For this review, take the finished solid that the model builds, in its own axes (mm). Face numbers are marked on the shaded views. A direction names the side the tool comes from. Give positions to 0.01 mm unless a question says otherwise; leave off trailing zeros. Order: outer loops, then holes, each group sorted by start corner. A loop starts at its lowest first (then second) coordinate and runs counter-clockwise, first axis right, second up. Notation, with made-up numbers: (71.5, 48) -> (101.5, 48) arc R23 ccw to (101.5, 86) -> close; hole circle Ø1 at (7, 15.25). An arc over 180 degrees is marked (long way). Use CSV: the item, a comma, the result in double quotes. Start each with the question number.
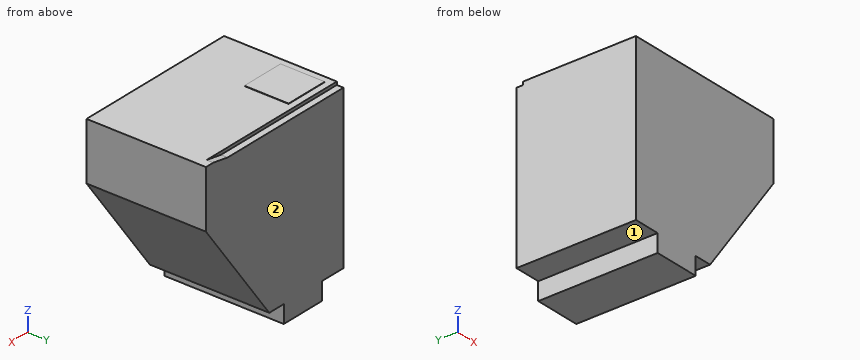
Solid Edge part; units mm, degrees
sketch "Sketch1" plane through (33.766, 0, 12.7127) normal (0, -1, 0) x (1, 0, 0)
  line L0 (-12.25, 0.75) -> (-21, -11.25)
  line L1 (-12.25, 7.25) -> (-12.25, 0.75)
  line L2 (-31.25, 7.25) -> (-12.25, 7.25)
  line L3 (-31.25, 7.25) -> (-31.25, -11.25)
  line L4 (-31.25, -11.25) -> (-28.25, -11.25)
  line L5 (-28.25, -11.25) -> (-28.25, -13.25)
  line L6 (-28.25, -13.25) -> (-23, -13.25)
  line L7 (-23, -13.25) -> (-23, -11.25)
  line L8 (-23, -11.25) -> (-21, -11.25)
extrude "Protrusion1" add sketch "Sketch1" along normal blind 13.5
sketch "Sketch2" plane through (12.016, -6.75, 19.9627) normal (0, 0, 1) x (1, 0, 0)
  line L0 (-9.5, 6.75) -> (6.5, 6.75)
  line L1 (6.5, 6.75) -> (6.5, 6)
  line L2 (6.5, 6) -> (-9.5, 6)
  line L3 (-9.5, 6) -> (-9.5, 6.75)
extrude "ExtrudedCutout_1" cut sketch "Sketch2" against normal blind 0.35
sketch "Sketch3" plane through (12.016, 0, 9.7127) normal (0, 1, 0) x (-1, 0, 0)
  line L0 (-8.5, 10.25) -> (-6.5, 9.9)
  line L1 (-6.5, 9.9) -> (-6.5, 10.25)
  line L2 (-6.5, 10.25) -> (-8.5, 10.25)
extrude "ExtrudedCutout_2" cut sketch "Sketch3" against normal blind 0.75
sketch "Sketch4" plane through (12.016, -6.75, 19.9627) normal (0, 0, 1) x (0, -1, 0)
  line L0 (-5.25, -8.75) -> (-5.25, -3.75)
  line L1 (-5.25, -3.75) -> (-0.25, -3.75)
  line L2 (-0.25, -3.75) -> (-0.25, -8.75)
  line L3 (-0.25, -8.75) -> (-5.25, -8.75)
extrude "ExtrudedProtrusion_2" add sketch "Sketch4" along normal blind 0.035
properties material "Stainless Steel, 420"
1. Clearance check with flat-ended pins moving along their axes: P1, Ø1, axis at y = -5.5, z = 0.5, coming from the +X side; P2, Ø0.6, axis at y = -6.5, z = 0, coming from the -X side; P3, Ø1.6, axis at x = 12, y = -9, coming from the -Z side. State where each tip first meets the part, or that it passes through.
2. Consider section C-C (y = -7.5). State the section outline as (x, z) points, plus the area to 4 significant figures.
3. Consider section D-D (z = 6). State the section outline as (x, y) points, plus the area to 3 significant figures.
4. For the marked faces 1 and 2, list the 3-axis set-ups (+Z, -Z, +X, -X, +Y, -Y) from which the entire face can be reached by the end or side of a thin tool; tool diameter is ignored.
5. To check wall thickness, follow L1, parallel to Z at x = 6.25, y = -7.25; L2, parallel to Z at x = 4, y = -5.5; L3, parallel to X at y = -8.75, z = 8.5. State the ranges of each line that lie inside material, in increasing order. Write a range as [from, to].
Answer list:
1,P1,"x = 10.77"
1,P2,"x = 5.52"
1,P3,"z = 1.46"
2,outline,"(2.52, 1.46) -> (5.52, 1.46) -> (5.52, -0.54) -> (10.77, -0.54) -> (10.77, 1.46) -> (12.77, 1.46) -> (21.52, 13.46) -> (21.52, 19.96) -> (2.52, 19.96) -> close"
2,area,"309.5 mm2"
3,outline,"(2.52, -13.5) -> (16.07, -13.5) -> (16.07, 0) -> (2.52, 0) -> close"
3,area,"183 mm2"
4,face 1,"-Z, -X, +Y, -Y"
4,face 2,"+Z, -Z, +X, -X, +Y"
5,L1,"[-0.54, 19.96]"
5,L2,"[1.46, 20]"
5,L3,"[2.52, 17.9]"
